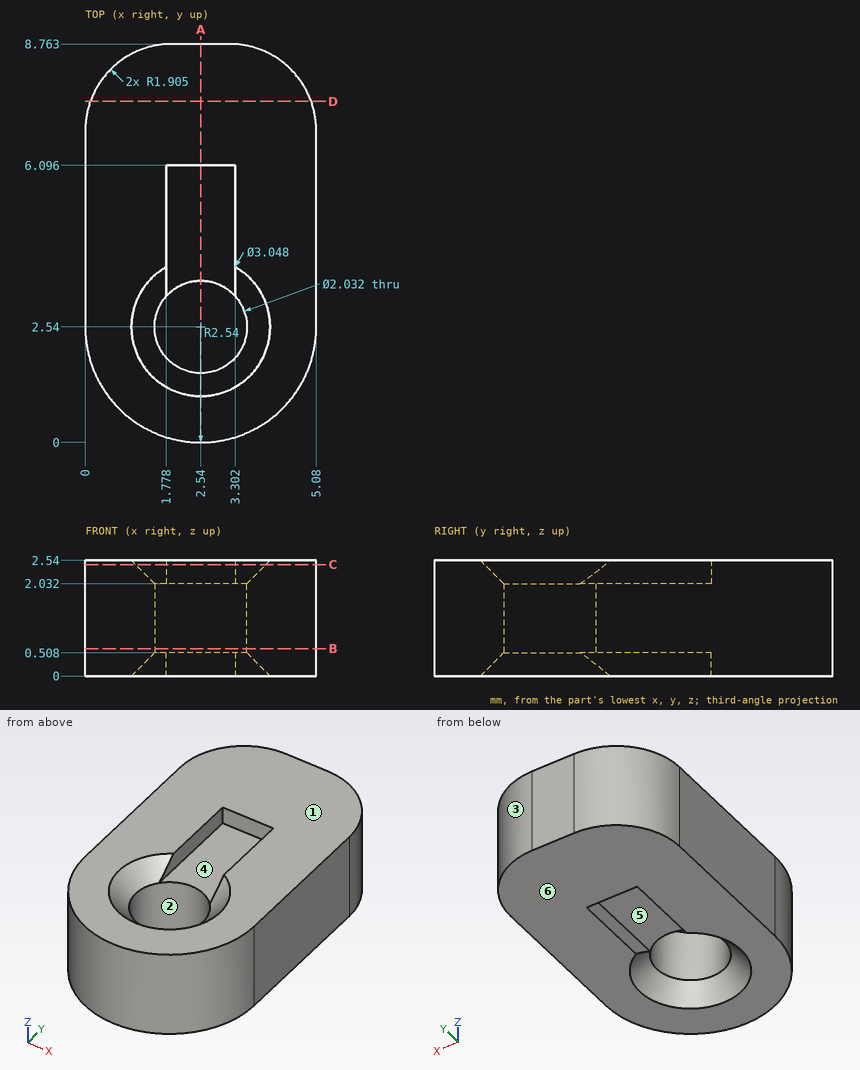
Here's the drawing with two shaded views (mm, measured from the low corner). I have some questions. A direction names the side the tool comes from. Coordinates: 2 decimals unless noted, no trailing zeros. Loops run counter-clockwise (first coordinate to the right, second up) from the corner with the lowest first, then second, coordinate; pieces in that order, holes last. Notation, with made-up numbers: M 77,42 L 112,42 A11 ccw 112,62 Z; hole C 33,36 d4. An arc over 180 degrees is marked long. Answer as CSV lines item,"result". Start each with the question number.
1. For pin 1 Ø0.5 at (x, y) = (2.5, 5.5) entering from -Z, with a flat end and sliding along its axis, tell me the tip position at first contact or that it passes through.
2. For the marked faces 4, 5 and 6, which set-ups out of +Z, -Z, +X, -X, +Y, -Y let a thin tool reach every point of the face, with its end or its side?
3. Suppose I cut it at A-A, the plane x = 2.54. List the corners of the cut face in (y, z) for me, plus the area to 3 significant figures.
4. Suppose I cut it at B-B, the plane z = 0.6. List the corners of the cut face in (x, y) for me (3 decimals), plus the area to 3 significant figures.
5. Thinking about a two-plate mould opening in Y: for the marked faces 1, 2 and 3, which applies, +Y half, -Y half, draft (parallel to the pull), parting line (faces both ways), or undercut?
6. If I drill on probe 1 along Y at (x, z) = (2.54, 1.35); probe 2 along X at (y, z) = (2.5, 0.6); probe 3 along Y at (x, z) = (2.1, 0.45), over which ranges is the centre line in solid material (lowest first)? Write a range as [from, to].
7. Suppose I cut it at C-C, the plane z = 2.45. List the corners of the cut face in (x, y) for me (3 decimals), plus the area to 3 significant figures.
8. Suppose I cut it at D-D, the plane y = 7.5. List the corners of the cut face in (x, z) for me, plus the area to 3 significant figures.
Output:
1,pin 1,"stops at z = 0.51"
2,face 4,"+Z"
2,face 5,"-Z"
2,face 6,"-Z, +X, -X, +Y, -Y"
3,outline,"M 0,0 L 1.02,0 L 1.52,0.51 L 1.52,2.03 L 1.02,2.54 L 0,2.54 Z; M 3.56,0.51 L 6.1,0.51 L 6.1,0 L 8.76,0 L 8.76,2.54 L 6.1,2.54 L 6.1,2.03 L 3.56,2.03 Z"
3,area,"14.3 mm^2"
4,outline,"M 0,2.54 A2.54 ccw 5.08,2.54 L 5.08,6.858 A1.905 ccw 3.175,8.763 L 1.905,8.763 A1.905 ccw 0,6.858 Z; hole C 2.54,2.54 d2.032"
4,area,"36.9 mm^2"
5,face 1,"draft"
5,face 2,"undercut"
5,face 3,"+Y half"
6,probe 1,"y = [0, 1.52], [3.56, 8.76]"
6,probe 2,"x = [0, 1.52], [3.56, 5.08]"
6,probe 3,"y = [0.04, 1.56], [6.1, 8.76]"
7,outline,"M 0,2.54 A2.54 ccw 5.08,2.54 L 5.08,6.858 A1.905 ccw 3.175,8.763 L 1.905,8.763 A1.905 ccw 0,6.858 Z; hole M 1.778,3.755 A1.434 ccw long 3.302,3.755 L 3.302,6.096 L 1.778,6.096 Z"
7,area,"30.4 mm^2"
8,outline,"M 0.11,0 L 4.97,0 L 4.97,2.54 L 0.11,2.54 Z"
8,area,"12.3 mm^2"
